from build123d import *

# Parameters (mm, degrees)
CYLINDER008_R     = 2
CYLINDER008_DEPTH = 20
CYLINDER007_R     = 2
CYLINDER007_DEPTH = 20
CYLINDER006_R     = 5
CYLINDER006_DEPTH = 20
BOX002_W          = 105
BOX002_H          = 65
BOX002_DEPTH      = 20
BOX001_W          = 115
BOX001_H          = 75
BOX001_DEPTH      = 10
FILLET_R          = 2
CYLINDER003_R     = 2
CYLINDER003_DEPTH = 10
CYLINDER002_R     = 2
CYLINDER002_DEPTH = 10
CYLINDER004_R     = 2
CYLINDER004_DEPTH = 10
CYLINDER005_R     = 2
CYLINDER005_DEPTH = 10
CYLINDER001_R     = 2
CYLINDER001_DEPTH = 10
CYLINDER_R        = 2
CYLINDER_DEPTH    = 10
BOX_W             = 140
BOX_H             = 100
BOX_DEPTH         = 4
CHAMFER_SIZE      = 1.5
CHAMFER001_SIZE   = 2
FILLET001_R       = 4
FILLET002_R       = 4
CHAMFER002_SIZE   = 1.5


with BuildPart() as cylinder008:
    # Cylinder008 → Cylinder008 (new body)
    with BuildSketch(Plane(origin=(70, 6, 0), x_dir=(1, 0, 0), z_dir=(0, 0, 1))):
        Circle(CYLINDER008_R)
    extrude(amount=CYLINDER008_DEPTH)


with BuildPart() as cylinder007:
    # Cylinder007 → Cylinder007 (new body)
    with BuildSketch(Plane(origin=(70, 94, 0), x_dir=(1, 0, 0), z_dir=(0, 0, 1))):
        Circle(CYLINDER007_R)
    extrude(amount=CYLINDER007_DEPTH)


with BuildPart() as cylinder006:
    # Cylinder006 → Cylinder006 (new body)
    with BuildSketch(Plane(origin=(70, 50, -5), x_dir=(1, 0, 0), z_dir=(0, 0, 1))):
        Circle(CYLINDER006_R)
    extrude(amount=CYLINDER006_DEPTH)


with BuildPart() as cube002:
    # Box002 → Box002 (new body)
    with BuildSketch(Plane(origin=(17.5, 17.5, 3), x_dir=(1, 0, 0), z_dir=(0, 0, 1))):
        with Locations((52.5, 32.5)):
            Rectangle(BOX002_W, BOX002_H)
    extrude(amount=BOX002_DEPTH)


with BuildPart() as fillet_body:
    # Box001 → Box001 (new body)
    with BuildSketch(Plane(origin=(12.5, 12.5, 0), x_dir=(1, 0, 0), z_dir=(0, 0, 1))):
        with Locations((57.5, 37.5)):
            Rectangle(BOX001_W, BOX001_H)
    extrude(amount=BOX001_DEPTH)

    # Fillet
    fillet_edges = [fillet_body.edges().sort_by_distance(p)[0] for p in [
        (12.5, 50, 0),
        (127.5, 50, 0),
        (70, 12.5, 0),
        (70, 87.5, 0),
    ]]
    fillet(fillet_edges, radius=FILLET_R)


with BuildPart() as cylinder003:
    # Cylinder003 → Cylinder003 (new body)
    with BuildSketch(Plane(origin=(6, 94, 0), x_dir=(1, 0, 0), z_dir=(0, 0, 1))):
        Circle(CYLINDER003_R)
    extrude(amount=CYLINDER003_DEPTH)


with BuildPart() as cylinder002:
    # Cylinder002 → Cylinder002 (new body)
    with BuildSketch(Plane(origin=(6, 50, 0), x_dir=(1, 0, 0), z_dir=(0, 0, 1))):
        Circle(CYLINDER002_R)
    extrude(amount=CYLINDER002_DEPTH)


with BuildPart() as cylinder004:
    # Cylinder004 → Cylinder004 (new body)
    with BuildSketch(Plane(origin=(6, 6, 0), x_dir=(1, 0, 0), z_dir=(0, 0, 1))):
        Circle(CYLINDER004_R)
    extrude(amount=CYLINDER004_DEPTH)


with BuildPart() as cylinder005:
    # Cylinder005 → Cylinder005 (new body)
    with BuildSketch(Plane(origin=(134, 94, 0), x_dir=(1, 0, 0), z_dir=(0, 0, 1))):
        Circle(CYLINDER005_R)
    extrude(amount=CYLINDER005_DEPTH)


with BuildPart() as cylinder001:
    # Cylinder001 → Cylinder001 (new body)
    with BuildSketch(Plane(origin=(134, 50, 0), x_dir=(1, 0, 0), z_dir=(0, 0, 1))):
        Circle(CYLINDER001_R)
    extrude(amount=CYLINDER001_DEPTH)


with BuildPart() as cylinder:
    # Cylinder → Cylinder (new body)
    with BuildSketch(Plane(origin=(134, 6, 0), x_dir=(1, 0, 0), z_dir=(0, 0, 1))):
        Circle(CYLINDER_R)
    extrude(amount=CYLINDER_DEPTH)


with BuildPart() as chamfer002:
    # Box → Box (new body)
    with BuildSketch(Plane.XY):
        with Locations((70, 50)):
            Rectangle(BOX_W, BOX_H)
    extrude(amount=BOX_DEPTH)

    # Cut: cut Cylinder
    add(cylinder.part, mode=Mode.SUBTRACT)

    # Cut001: cut Cylinder001
    add(cylinder001.part, mode=Mode.SUBTRACT)

    # Cut002: cut Cylinder005
    add(cylinder005.part, mode=Mode.SUBTRACT)

    # Cut003: cut Cylinder004
    add(cylinder004.part, mode=Mode.SUBTRACT)

    # Cut004: cut Cylinder002
    add(cylinder002.part, mode=Mode.SUBTRACT)

    # Cut005: cut Cylinder003
    add(cylinder003.part, mode=Mode.SUBTRACT)


with BuildPart() as chamfer002_1:
    # Cut005 placement: moved
    add(chamfer002.part.moved(Location((0, 0, 10))))

    # Chamfer
    chamfer_edges = [chamfer002_1.edges().sort_by_distance(p)[0] for p in [
        (4, 50, 14),
        (4, 6, 14),
        (0, 50, 14),
        (70, 100, 14),
        (70, 0, 14),
        (140, 50, 14),
        (4, 94, 14),
        (132, 94, 14),
        (132, 50, 14),
        (132, 6, 14),
    ]]
    chamfer(chamfer_edges, length=CHAMFER_SIZE)

    # Fusion: union Fillet body
    add(fillet_body.part)

    # Cut006: cut Cube002
    add(cube002.part, mode=Mode.SUBTRACT)

    # Cut007: cut Cylinder006
    add(cylinder006.part, mode=Mode.SUBTRACT)

    # Chamfer001
    chamfer001_edges = [chamfer002_1.edges().sort_by_distance(p)[0] for p in [
        (122.5, 50, 14),
        (70, 17.5, 14),
        (17.5, 50, 14),
        (70, 82.5, 14),
    ]]
    chamfer(chamfer001_edges, length=CHAMFER001_SIZE)

    # Fillet001
    fillet001_edges = [chamfer002_1.edges().sort_by_distance(p)[0] for p in [
        (140, 0, 11.25),
        (140, 100, 11.25),
    ]]
    fillet(fillet001_edges, radius=FILLET001_R)

    # Fillet002
    fillet002_edges = [chamfer002_1.edges().sort_by_distance(p)[0] for p in [
        (0, 0, 11.25),
        (0, 100, 11.25),
    ]]
    fillet(fillet002_edges, radius=FILLET002_R)

    # Cut008: cut Cylinder007
    add(cylinder007.part, mode=Mode.SUBTRACT)

    # Cut009: cut Cylinder008
    add(cylinder008.part, mode=Mode.SUBTRACT)

    # Chamfer002
    chamfer002_edges = [chamfer002_1.edges().sort_by_distance(p)[0] for p in [
        (68, 6, 14),
        (68, 94, 14),
    ]]
    chamfer(chamfer002_edges, length=CHAMFER002_SIZE)


solid = chamfer002_1.part
CAD build for the part. Positions are in the model's coordinates, mm. A direction names the side the tool comes from. Give positions to 0.01 mm unless a question says otherwise; leave off trailing zeros. Order: outer loops, then holes, each group sorted by start corner. A loop starts at its lowest first (then second) coordinate and runs counter-clockwise, first axis right, second up. Notation, with made-up numbers: (87.25, -38) -> (91.25, -38) arc R13 ccw to (91.25, -20) -> close; hole circle Ø2 at (78, 75.25). An arc over 180 degrees is marked (long way). Return JSON: item names as keys, results as strings.
Q1. Saw through at A-A (x = 70). Count the separate pieces of the cut face and the enclosed holes in it, then the cut area to 3 significant figures.
Working result:
{"separate pieces": "4", "enclosed holes": "0", "area": "361 mm²"}
Q2. Mould opens along Y. For faces 1 (the face through (69, 58, 3)), 2 (the face through (127.5, 49, 6)), 3 (the face through (69, 87.5, 6)), 4 (the face through (4.526, 7.352, 11.232)) say: pulls with the +Y half, pulls with the -Y half, needs draft (parallel to the pull), parting line crosses it, or undercut.
Working result:
{"face 1": "undercut", "face 2": "needs draft", "face 3": "pulls with the +Y half", "face 4": "undercut"}
Q3. Saw through at C-C (y = 6). Write the cut outline in (x, z), then the cut area to 3 significant figures.
Working result:
{"outline": "(0, 10) -> (4, 10) -> (4, 12.5) -> (2.5, 14) -> (1.5, 14) -> (0, 12.5) -> close; (8, 10) -> (68, 10) -> (68, 12.5) -> (66.5, 14) -> (9.5, 14) -> (8, 12.5) -> close; (72, 10) -> (132, 10) -> (132, 12.5) -> (130.5, 14) -> (73.5, 14) -> (72, 12.5) -> close; (136, 10) -> (140, 10) -> (140, 12.5) -> (138.5, 14) -> (137.5, 14) -> (136, 12.5) -> close", "area": "503 mm²"}
Q4. Flat gauge pins, fed straight in: pin 1 (6.5 mm diameter, centred on x = 70, y = 6, fed in from +Z); pin 2 (3 mm diameter, centred on x = 134, y = 50, fed in from +Z); pin 3 (6.5 mm diameter, centred on x = 71, z = 5, fed in from -Y); pin 4 (2.5 mm diameter, centred on x = 80, z = 7, fed in from +Y). Where does each tip first touch, or does it go through?
Working result:
{"pin 1": "z = 13.75", "pin 2": "through", "pin 3": "y = 12.5", "pin 4": "y = 87.5"}
Q5. Drill centre lines: line 1 (X direction, y = 6, z = 12.05); line 2 (X direction, y = 50, z = 11.05); line 3 (Y direction, x = 6, z = 11.25). Where is each one in solid material? Low to high.
Working result:
{"line 1": "0 to 4, 8 to 68, 72 to 132, 136 to 140", "line 2": "0 to 4, 8 to 17.5, 122.5 to 132, 136 to 140", "line 3": "0 to 4, 8 to 48, 52 to 92, 96 to 100"}
Q6. Saw through at B-B (z = 6.5). Write the cut outline in (x, y).
Working result:
{"outline": "(12.5, 12.5) -> (127.5, 12.5) -> (127.5, 87.5) -> (12.5, 87.5) -> close; hole (17.5, 17.5) -> (122.5, 17.5) -> (122.5, 82.5) -> (17.5, 82.5) -> close"}
Q7. Saw through at D-D (y = 60). Write the cut outline in (x, z).
Working result:
{"outline": "(0, 10) -> (12.5, 10) -> (12.5, 2) arc R2 ccw to (14.5, 0) -> (125.5, 0) arc R2 ccw to (127.5, 2) -> (127.5, 10) -> (140, 10) -> (140, 12.5) -> (138.5, 14) -> (124.5, 14) -> (122.5, 12) -> (122.5, 3) -> (17.5, 3) -> (17.5, 12) -> (15.5, 14) -> (1.5, 14) -> (0, 12.5) -> close"}
Q8. Which spindle directions (+Z, -Z, +X, -X, +Y, -Y) get a long thin tool onto all of the face, cutting with end or side? Do faces 5 (the face through (69, 12.5, 6)), 6 (the face through (73, 54, 1)), 7 (the face through (69, 17.5, 7)). Say none if no direction does.
Working result:
{"face 5": "-Z, +X, -X, -Y", "face 6": "+Z, -Z", "face 7": "+Z"}
